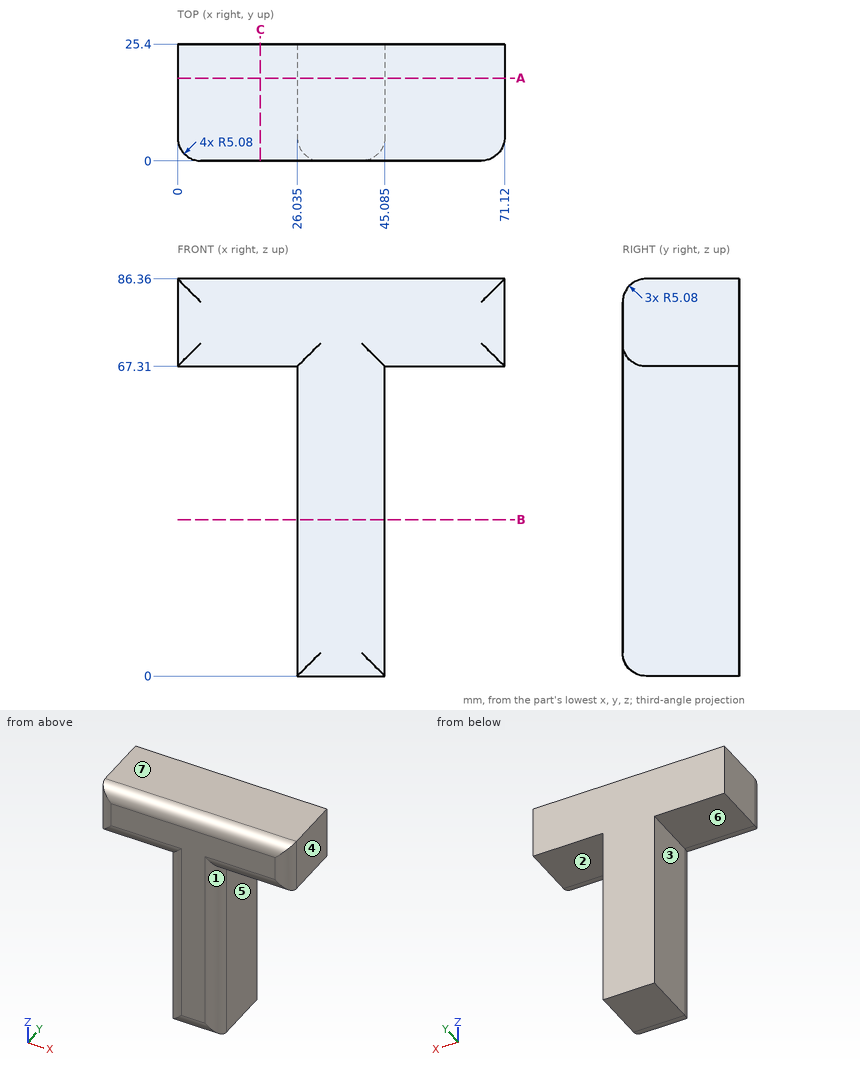
Could you check a few things on this drawing? It's one solid part, dimensions in mm from its lowest x, y, z. A direction names the side the tool comes from. Give positions to 0.01 mm unless a question says otherwise; leave off trailing zeros. Write each loop counter-clockwise with the first axis right and the second up, starting at its lowest first coordinate (ties: lowest second). Pieces come first, ordered by that corner, then holes. Notation, with made-up numbers: (48, 24.5) -> (82, 24.5) arc R19 cw to (82, 32.5) -> close; hole circle Ø11 at (-21, 44). An arc over 180 degrees is marked (long way). Answer as a JSON object with one key per item and string values.
Q1. Which directions (+Z, -Z, +X, -X, +Y, -Y) give clear straight access to the entire face, cutting with the end or side of a thin tool? Please do the marked faces 1, 2, 3 and 4.
Taken from the geometry:
{"face 1": "-Z, +X, -Y", "face 2": "-Z, +X, +Y, -Y", "face 3": "-Z, -X, +Y, -Y", "face 4": "+Z, -Z, +X, +Y, -Y"}
Q2. Suppose I cut it at C-C on x = 18. Write out the boundary of the cut face in (y, z), then the cut area to 3 significant figures.
Taken from the geometry:
{"outline": "(0, 72.39) arc R5.08 ccw to (5.08, 67.31) -> (25.4, 67.31) -> (25.4, 86.36) -> (5.08, 86.36) arc R5.08 ccw to (0, 81.28) -> close", "area": "473 mm²"}
Q3. Will these pins go through, and if not, where does the flat tip stop? pin 1 Ø6 at (x, z) = (47, 37) entering from -Y; pin 2 Ø10 at (y, z) = (10.5, 27) entering from -X (3 decimals); pin 3 Ø1 at (x, z) = (9.5, 68.5) entering from -Y.
Taken from the geometry:
{"pin 1": "stops at y = 1.94", "pin 2": "stops at x = 26.035", "pin 3": "stops at y = 1.3"}
Q4. Suppose I cut it at B-B on z = 34. Write out the boundary of the cut face in (x, y) (3 decimals), then the cut area to 3 significant figures.
Taken from the geometry:
{"outline": "(26.035, 5.08) arc R5.08 ccw to (31.115, 0) -> (40.005, 0) arc R5.08 ccw to (45.085, 5.08) -> (45.085, 25.4) -> (26.035, 25.4) -> close", "area": "473 mm²"}
Q5. Suppose I cut it at A-A on y = 18. Write out the boundary of the cut face in (x, z) (3 decimals).
Taken from the geometry:
{"outline": "(0, 67.31) -> (26.035, 67.31) -> (26.035, 0) -> (45.085, 0) -> (45.085, 67.31) -> (71.12, 67.31) -> (71.12, 86.36) -> (0, 86.36) -> close"}
Q6. We'd pull the mould along Z, two halves only. Please class the marked faces 5, 6 and 7: released by +Z, released by -Z, zero draft, split by the parting line, or undercut.
Taken from the geometry:
{"face 5": "zero draft", "face 6": "released by -Z", "face 7": "released by +Z"}
Q7. Please list where these lines run through material, in increasing order: L1, parallel to Z at x = 3.5, y = 11; L2, parallel to X at y = 12, z = 15.5 (3 decimals); L3, parallel to X at y = 2, z = 40.
Taken from the geometry:
{"L1": "z = 67.31 to 86.36", "L2": "x = 26.035 to 45.085", "L3": "x = 27.08 to 44.04"}
